from build123d import *

# Parameters (mm, degrees)
SKETCH1_R           = 2.3
BOSS_EXTRUDE1_DEPTH = 15
SKETCH2_W           = 4.6
SKETCH2_H           = 7
BOSS_EXTRUDE2_DEPTH = 3
CUT_EXTRUDE1_DEPTH  = 4.6


with BuildPart() as part:
    # Sketch1 → Boss-Extrude1 (new body)
    with BuildSketch(Plane.XY):
        Circle(SKETCH1_R)
    extrude(amount=BOSS_EXTRUDE1_DEPTH)

    # Sketch2 → Boss-Extrude2 (add)
    with BuildSketch(Plane(origin=(0, 0, 0), x_dir=(-1, 0, 0), z_dir=(0, 0, -1))):
        Rectangle(SKETCH2_W, SKETCH2_H)
    extrude(amount=BOSS_EXTRUDE2_DEPTH)

    # Sketch3 → Cut-Extrude1 (cut)
    with BuildSketch(Plane(origin=(2.3, 0, 0), x_dir=(0, 0, -1), z_dir=(1, 0, 0))):
        with BuildLine():
            Line((1.2, -3.5), (3, -3.5))
            Line((3, -3.5), (3, 3.5))
            Line((3, 3.5), (2.011534301, 3.5))
            add(Edge.make_bspline(
                [(1.2, -3.5), (2.267514736, -1.334400874), (2.08240034, 1.182388913), (2.011534301, 3.5)],
                knots=[0, 0, 0, 0, 1, 1, 1, 1], degree=3))
        make_face()
    extrude(amount=-CUT_EXTRUDE1_DEPTH, mode=Mode.SUBTRACT)


solid = part.part
Geometry check sheet. Reference: the model listing, model coordinates, mm. A direction names the side the tool comes from. Round coordinates to 2 decimals unless told otherwise and drop trailing zeros. Write each loop counter-clockwise with the first axis right and the second up, starting at its lowest first coordinate (ties: lowest second). Pieces come first, ordered by that corner, then holes. Notation, with made-up numbers: (22, 5.5) -> (70, 5.5) arc R35 ccw to (70, 40.5) -> close; hole circle Ø7 at (-39.75, 58.5). An arc over 180 degrees is marked (long way). One line per item, written item: value. Start each with the question number.
(1) Go/stop test with a flat-tipped pin: pin 1 Ø2 at (x, y) = (1, -2) entering from -Z. Record where the tip stops, or that it passes through.
(2) Scan lines: line 1 (Z direction, x = 0.95, y = -3); line 2 (Y direction, x = -1.7, z = 6); line 3 (X direction, y = 1, z = 12). Record each from-to range of solid material in increasing order. Write a range as [from, to].
(3) Cross-section at A-A, the plane z = 1.5. Record the cut outline in (x, y).
(4) Access from +Z, -Z, +X, -X, +Y, -Y to the whole of each face (thin tool, end or side, straight path). Record for faces 1 (the cylindrical face through (-1.825, -1.4, 7.395)), 2 (the flat face through (0, -3.5, -1)), 3 (the flat face through (0, -3, 0)), 4 (the flat face through (0, 3, 0)).
Answer:
1. pin 1: z = -1.94
2. line 1: [-1.42, 0]
2. line 2: [-1.55, 1.55]
2. line 3: [-2.07, 2.07]
3. outline: circle Ø4.6 at (0, 0)
4. face 1: +Z
4. face 2: +Z, -Z, +X, -X, -Y
4. face 3: +Z, -Y
4. face 4: +Z, +Y
